Source: CAD feature listing. Evaluate the final solid. Frame: model axes, mm. Round coordinates to 2 decimals unless told otherwise and drop trailing zeros. Order: outer loops, then holes, each group sorted by start corner. A loop starts at its lowest first (then second) coordinate and runs counter-clockwise, first axis right, second up. Notation, with made-up numbers: (3.25, 27.25) -> (21.25, 27.25) arc R19 cw to (21.25, 35.25) -> close; hole circle Ø3 at (68, 35). An arc over 180 degrees is marked (long way). Answer as CSV lines item,"result". Start each with the question number.
(1) Line query: line 1 along X through (y, z) = (-0.8, -159) (3 decimals); line 2 along X through (y, z) = (-0.6, -152); line 3 along X through (y, z) = (-1, 78.5). Output: solid intervals per line, ascending. Write a range as from..to.
(2) Section query B-B (z = -153). Output: boundary loops of the cut face in (x, y), plus the area to 3 significant figures.
(3) Section query A-A (y = -1.5). Output: boundary loops of the cut face in (x, z).
(4) Contact query for a flat-ended pin moving along its axis: P1, Ø8.5, axis at x = -115, z = 173, coming from the -Y side. Output: stop coordinate, or through.
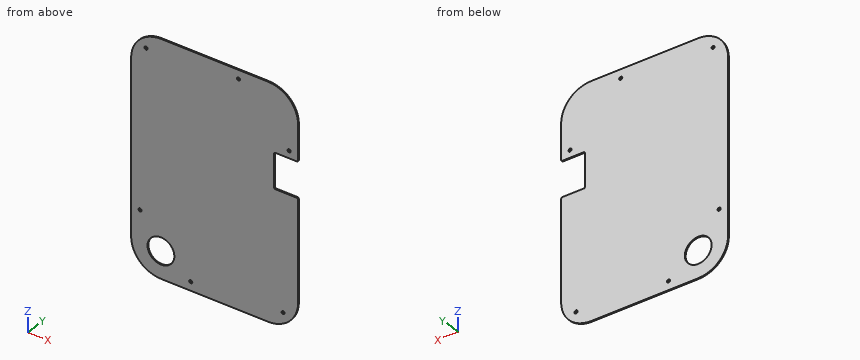
```python
from build123d import *

# Parameters (mm, degrees)
SKETCH1_W             = 280
SKETCH1_H             = 396
BASE_FLANGE1_DEPTH    = 2
BREAK_CORNER1_START   = -2
BREAK_CORNER1_DEPTH   = 2
SKETCH2_R             = 22.5
CUT_EXTRUDE1_DEPTH    = 243.503608221
SKETCH3_R             = 2.6
CUT_EXTRUDE2_DEPTH    = 243.503608221
SKETCH4_W             = 40
SKETCH4_H             = 60
CUT_EXTRUDE3_DEPTH    = 243.503608221
BREAK_CORNER2_START   = -2
BREAK_CORNER2_DEPTH   = 2
BREAK_CORNER2_2_DEPTH = 2


# Read off the part's stored shape, not the designer's step: Break-Corner1, Break-Corner2
# Sheet-metal steps are written as plain solids
with BuildPart() as part:
    # Sketch1 → Base-Flange1 (new body)
    with BuildSketch(Plane(origin=(0, 0, 0), x_dir=(1, 0, 0), z_dir=(0, 1, 0))):
        Rectangle(SKETCH1_W, SKETCH1_H)
    extrude(amount=-BASE_FLANGE1_DEPTH)

    # Break-Corner1 outline → Break-Corner1 (cut)
    with BuildSketch(Plane(origin=(0, 0, 0), x_dir=(1, 0, 0), z_dir=(0, 1, 0)).offset(BREAK_CORNER1_START)):
        with BuildLine():
            ThreePointArc((-140, 148), (-125.355339059, 183.355339059), (-90, 198))
            Line((-90, 198), (-140, 198))
            Line((-140, 198), (-140, 148))
        make_face()
        with BuildLine():
            Line((140, 198), (90, 198))
            ThreePointArc((90, 198), (125.355339059, 183.355339059), (140, 148))
            Line((140, 148), (140, 198))
        make_face()
        with BuildLine():
            ThreePointArc((-90, -198), (-125.355339059, -183.355339059), (-140, -148))
            Line((-140, -148), (-140, -198))
            Line((-140, -198), (-90, -198))
        make_face()
        with BuildLine():
            Line((140, -198), (140, -148))
            ThreePointArc((140, -148), (125.355339059, -183.355339059), (90, -198))
            Line((90, -198), (140, -198))
        make_face()
    extrude(amount=BREAK_CORNER1_DEPTH, mode=Mode.SUBTRACT)

    # Sketch2 → Cut-Extrude1 (cut, through all)
    with BuildSketch(Plane(origin=(0, 0, 0), x_dir=(1, 0, 0), z_dir=(0, 1, 0))):
        with Locations(Location((-90, 152, 0), (0, 0, 270))):
            Circle(SKETCH2_R)
    extrude(amount=-CUT_EXTRUDE1_DEPTH, mode=Mode.SUBTRACT)

    # Sketch3 → Cut-Extrude2 (cut, through all)
    with BuildSketch(Plane(origin=(0, 0, 0), x_dir=(1, 0, 0), z_dir=(0, 1, 0))):
        with Locations(Location((-40, 183, 0), (0, 0, 270))):
            Circle(SKETCH3_R)
        with Locations(Location((-125, 98, 0), (0, 0, 270))):
            Circle(SKETCH3_R)
        with Locations(Location((125, -98, 0), (0, 0, 270))):
            Circle(SKETCH3_R)
        with Locations(Location((40, -183, 0), (0, 0, 270))):
            Circle(SKETCH3_R)
        with Locations(Location((-115, -173, 0), (0, 0, 270))):
            Circle(SKETCH3_R)
        with Locations(Location((115, 173, 0), (0, 0, 270))):
            Circle(SKETCH3_R)
    extrude(amount=-CUT_EXTRUDE2_DEPTH, mode=Mode.SUBTRACT)

    # Sketch4 → Cut-Extrude3 (cut, through all)
    with BuildSketch(Plane(origin=(0, 0, 0), x_dir=(1, 0, 0), z_dir=(0, 1, 0))):
        with Locations((120, -55.5)):
            Rectangle(SKETCH4_W, SKETCH4_H)
    extrude(amount=-CUT_EXTRUDE3_DEPTH, mode=Mode.SUBTRACT)

    # Break-Corner2 outline → Break-Corner2 (cut)
    with BuildSketch(Plane(origin=(0, 0, 0), x_dir=(1, 0, 0), z_dir=(0, 1, 0)).offset(BREAK_CORNER2_START)):
        with BuildLine():
            Line((140, -85.5), (138, -85.5))
            ThreePointArc((138, -85.5), (139.414213562, -86.085786438), (140, -87.5))
            Line((140, -87.5), (140, -85.5))
        make_face()
        with BuildLine():
            ThreePointArc((140, -23.5), (139.414213562, -24.914213562), (138, -25.5))
            Line((138, -25.5), (140, -25.5))
            Line((140, -25.5), (140, -23.5))
        make_face()
    extrude(amount=BREAK_CORNER2_DEPTH, mode=Mode.SUBTRACT)

    # Break-Corner2 2 outline → Break-Corner2 2 (add)
    with BuildSketch(Plane(origin=(0, 0, 0), x_dir=(1, 0, 0), z_dir=(0, 1, 0)).offset(BREAK_CORNER2_START)):
        with BuildLine():
            Line((100, -25.5), (100, -27.5))
            ThreePointArc((100, -27.5), (100.585786438, -26.085786438), (102, -25.5))
            Line((102, -25.5), (100, -25.5))
        make_face()
        with BuildLine():
            ThreePointArc((102, -85.5), (100.585786438, -84.914213562), (100, -83.5))
            Line((100, -83.5), (100, -85.5))
            Line((100, -85.5), (102, -85.5))
        make_face()
    extrude(amount=BREAK_CORNER2_2_DEPTH)


solid = part.part
```
Answer block:
1,line 1,"-138.775..-111.383, -68.617..138.775"
1,line 2,"-139.84..-112.5, -67.5..139.84"
1,line 3,"-140..100"
2,outline,"(-139.75, -2) -> (-112.48, -2) -> (-112.48, 0) -> (-139.75, 0) -> close; (-67.52, -2) -> (139.75, -2) -> (139.75, 0) -> (-67.52, 0) -> close"
2,area,"469 mm2"
3,outline,"(-140, -148) arc R50 ccw to (-90, -198) -> (90, -198) arc R50 ccw to (140, -148) -> (140, 23.5) arc R2 ccw to (138, 25.5) -> (102, 25.5) arc R2 cw to (100, 27.5) -> (100, 83.5) arc R2 cw to (102, 85.5) -> (138, 85.5) arc R2 ccw to (140, 87.5) -> (140, 148) arc R50 ccw to (90, 198) -> (-90, 198) arc R50 ccw to (-140, 148) -> close; hole circle Ø5.2 at (-125, -98); hole circle Ø5.2 at (-115, 173); hole circle Ø45 at (-90, -152); hole circle Ø5.2 at (-40, -183); hole circle Ø5.2 at (40, 183); hole circle Ø5.2 at (115, -173); hole circle Ø5.2 at (125, 98)"
4,P1,"y = -2"
